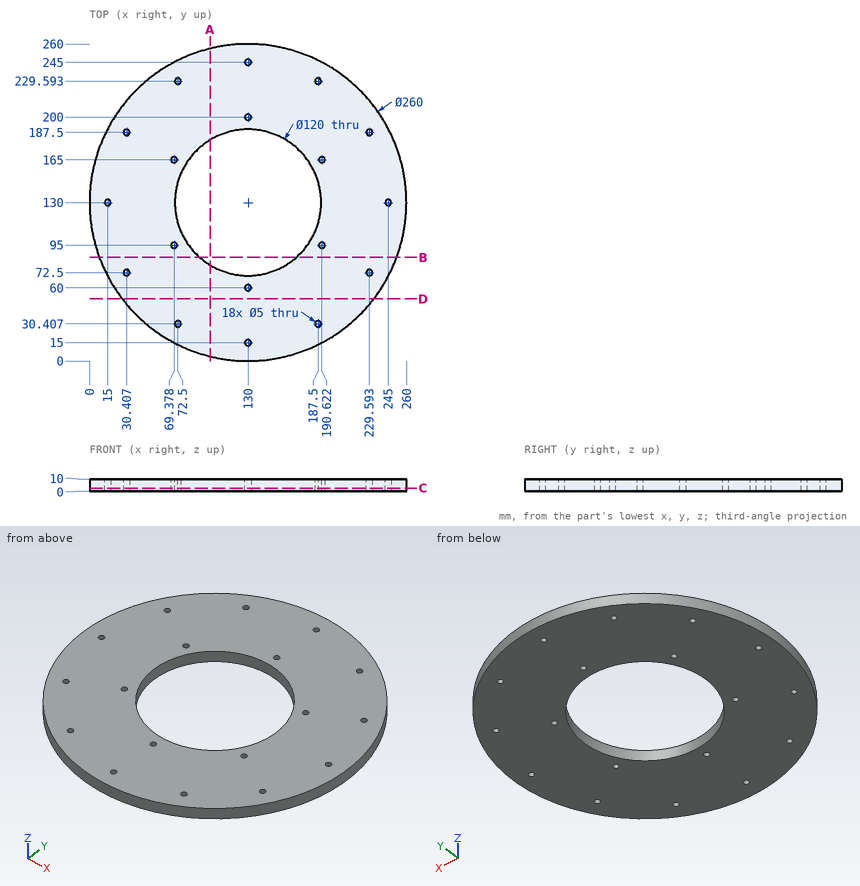
Input: dimensioned drawing with shaded views. Units: mm. Origin: part minimum x, y, z. Give positions to 0.01 mm unless a question says otherwise; leave off trailing zeros. Order: outer loops, then holes, each group sorted by start corner. A loop starts at its lowest first (then second) coordinate and runs counter-clockwise, first axis right, second up.
(1) Section query B-B (y = 85). Return the cut outline in (x, z), plus the area to 3 significant figures.
(2) Section query A-A (x = 99). Return the cut outline in (y, z).
(3) Section query D-D (y = 51). Return the cut outline in (x, z), plus the area to 4 significant figures.
(4) Contact query for flat-ended pins moving along their axis: P1, Ø6, axis at x = 187.5, y = 229.59, coming from the +Z side; P2, Ø1.5, axis at x = 220.5, z = 4, coming from the +Y side; P3, Ø4, axis at x = 69.38, y = 95, coming from the -Z side; P4, Ø1, axis at x = 142, z = 1, coming from the +Y side. Output: stop coordinate, or through.
(5) Section query C-C (z = 2.5). State how many separate pieces and enclosed holes the cut face has, plus the area to 3 significant figures.
(6) Material intervals for line 1 along Y through (x, z) = (130, 6.25); line 2 along X through (y, z) = (95, 8) (1 decimal); line 3 along Y through (x, z) = (43.5, 7.25) (1 decimal), sorted ascending.
Outcome:
1. outline: (8.04, 0) - (90.31, 0) - (90.31, 10) - (8.04, 10) - close; (169.69, 0) - (251.96, 0) - (251.96, 10) - (169.69, 10) - close
1. area: 1,650 mm2
2. outline: (3.75, 0) - (78.63, 0) - (78.63, 10) - (3.75, 10) - close; (181.37, 0) - (256.25, 0) - (256.25, 10) - (181.37, 10) - close
3. outline: (26.76, 0) - (233.24, 0) - (233.24, 10) - (26.76, 10) - close
3. area: 2,065 mm2
4. P1: stops at z = 10
4. P2: stops at y = 224.05
4. P3: passes through
4. P4: stops at y = 259.49
5. separate pieces: 1
5. enclosed holes: 19
5. area: 41,400 mm2
6. line 1: y = 0 to 12.5, 17.5 to 57.5, 62.5 to 70, 190 to 197.5, 202.5 to 242.5, 247.5 to 260
6. line 2: x = 4.8 to 66.9, 71.9 to 81.3, 178.7 to 188.1, 193.1 to 255.2
6. line 3: y = 33 to 227
